For this review, take the finished solid that the model builds, in its own axes (mm). A direction names the side the tool comes from. Coordinates: 2 decimals unless noted, no trailing zeros. Loops run counter-clockwise (first coordinate to the right, second up) from the corner with the lowest first, then second, coordinate; pieces in that order, holes last.
1. Take a section at D-D, the plane z = 4.5. State the section outline as (x, y) points, then the cut area to 3 significant figures.
2. Clearance check with flat-ended pins moving along their axes: P1, Ø0.5, axis at y = 2.5, z = 12, coming from the +X side; P2, Ø0.7, axis at y = -1, z = 9.5, coming from the -X side; P3, Ø4, axis at x = 0, z = 10, coming from the -Y side. State where each tip first meets the part, or that it passes through.
3. Take a section at C-C, the plane x = 1.25. State the section outline as (y, z) points.
4. Mouldability with a two-part tool opening along Z and no side actions: class faces 5 (the face through (1.46, -1.66, 12.47)), 6 (the face through (0, 0, 0)), 7 (the face through (-4.17, -1.7, 9.86)) as pulls with the +Z half, pulls with the -Z half, needs draft (parallel to the pull), parting line crosses it, or undercut.
5. Machinability: for faces 1 (the face through (2.94, 2, 10)), 2 (the face through (-2.94, 2, 10)), 3 (the face through (-1.46, -1.66, 7.53)), 4 (the face through (-1.29, 4.812, 12.024)), which of the approach directions +Z, -Z, +X, -X, +Y, -Y give a long, thin tool a straight path to every point of the face, cutting with its end or side? Answer none if there is none.
6. Take a section at B-B, the plane y = -1. State the section outline as (x, z) points.
7. To check wall thickness, follow probe 1 along Z at (x, y) = (0, 2.5); probe 2 along Z at (x, y) = (0, 4.75); probe 3 along X at (y, z) = (1, 10). State the ranges of each line that lie inside material, in increasing order.
8. Take a section at A-A, the plane z = 10. State the section outline as (x, y) points.
```python
from build123d import *

# Parameters (mm, degrees)
PAD_DEPTH       = 20
SKETCH001_R     = 1.6
POCKET_DEPTH    = 5.68
SKETCH002_R     = 2.4
SKETCH002_R_2   = 1.6
PAD001_DEPTH    = 4
SKETCH003_R     = 1.6
POCKET001_DEPTH = 2.4


with BuildPart() as part:
    # Sketch → Pad (new body)
    with BuildSketch(Plane.XY):
        Polygon((2.94, -2.84), (-2.94, -2.84), (-5.44, -0.52), (-5.44, 1.16), (-2.94, 1.16), (-2.94, 2.84), (2.94, 2.84), (2.94, 1.16), (5.44, 1.16), (5.44, -0.52), align=None)
    extrude(amount=PAD_DEPTH)

    # Sketch001 (on Face6 of Pad) → Pocket (cut)
    with BuildSketch(Plane(origin=(0, 2.84, 0), x_dir=(-1, 0, 0), z_dir=(0, 1, 0))):
        with Locations((0, 10)):
            Circle(SKETCH001_R)
    extrude(amount=-POCKET_DEPTH, mode=Mode.SUBTRACT)

    # Sketch002 (on Face11 of Pocket) → Pad001 (join)
    with BuildSketch(Plane(origin=(0, 2.84, 0), x_dir=(-1, 0, 0), z_dir=(0, 1, 0))):
        with Locations((0, 10)):
            Circle(SKETCH002_R)
        with Locations((0, 10)):
            Circle(SKETCH002_R_2, mode=Mode.SUBTRACT)
    extrude(amount=PAD001_DEPTH)

    # Sketch003 (on Face1 of Pad001) → Pocket001 (cut)
    with BuildSketch(Plane.XZ.offset(2.84)):
        Polygon((0, 6.686009), (2.87, 8.343005), (2.87, 11.656995), (0, 13.313991), (-2.87, 11.656995), (-2.87, 8.343005), align=None)
        with Locations((0, 10)):
            Circle(SKETCH003_R, mode=Mode.SUBTRACT)
    extrude(amount=-POCKET001_DEPTH, mode=Mode.SUBTRACT)


solid = part.part
```
Results list:
1. outline: (-5.44, -0.52) - (-2.94, -2.84) - (2.94, -2.84) - (5.44, -0.52) - (5.44, 1.16) - (2.94, 1.16) - (2.94, 2.84) - (-2.94, 2.84) - (-2.94, 1.16) - (-5.44, 1.16) - close
1. area: 47.6 mm2
2. P1: stops at x = 2.94
2. P2: stops at x = -5.3
2. P3: stops at y = -0.44
3. outline: (-2.84, 0) - (2.84, 0) - (2.84, 7.95) - (6.84, 7.95) - (6.84, 9) - (-0.44, 9) - (-0.44, 7.41) - (-2.84, 7.41) - close; (-2.84, 12.59) - (-0.44, 12.59) - (-0.44, 11) - (6.84, 11) - (6.84, 12.05) - (2.84, 12.05) - (2.84, 20) - (-2.84, 20) - close
4. face 5: undercut
4. face 6: pulls with the -Z half
4. face 7: needs draft
5. face 1: +Z, -Z, +X, +Y
5. face 2: +Z, -Z, -X, +Y
5. face 3: -Y
5. face 4: +Y
6. outline: (-4.92, 0) - (4.92, 0) - (4.92, 20) - (-4.92, 20) - close; hole (-2.87, 8.34) - (0, 6.69) - (2.87, 8.34) - (2.87, 11.66) - (0, 13.31) - (-2.87, 11.66) - close
7. probe 1: z = 0 to 8.4, 11.6 to 20
7. probe 2: z = 7.6 to 8.4, 11.6 to 12.4
7. probe 3: x = -5.44 to -1.6, 1.6 to 5.44
8. outline: (-5.44, -0.52) - (-2.94, -2.84) - (-2.87, -2.84) - (-2.87, -0.44) - (-1.6, -0.44) - (-1.6, 6.84) - (-2.4, 6.84) - (-2.4, 2.84) - (-2.94, 2.84) - (-2.94, 1.16) - (-5.44, 1.16) - close; (1.6, -0.44) - (2.87, -0.44) - (2.87, -2.84) - (2.94, -2.84) - (5.44, -0.52) - (5.44, 1.16) - (2.94, 1.16) - (2.94, 2.84) - (2.4, 2.84) - (2.4, 6.84) - (1.6, 6.84) - close
